Job drawing, mm, ordinate dimensions from the low corner. One solid piece. Give positions to 0.01 mm unless a question says otherwise; leave off trailing zeros. Write each loop counter-clockwise with the first axis right and the second up, starting at its lowest first coordinate (ties: lowest second). Pieces come first, ordered by that corner, then holes. Notation, with made-up numbers: (89.25, 48.25) - (139.25, 48.25) arc R22 cw to (139.25, 71.25) - close; hole circle Ø3 at (15, -37). An arc over 180 degrees is marked (long way). Put each result on its own line as item: value. Start each with the question number.
1. Cut at B-B on z = 65. List the corners of the cut face in (x, y), and give its area (3 significant figures).
2. Drop a flat-ended pin along its axis: pin 1 (4 mm diameter, centred on y = 3.5, z = 53.5, fed in from +X). Give the stop position or say it passes through.
3. Wall check: line 1 (Y direction, x = 0.4, z = 57); line 2 (Z direction, x = 0.35, y = 5.25). Give the ranges that are in metal, low to high.
4. Cut at A-A on x = 0.3. List the corners of the cut face in (y, z), and give its area (3 significant figures).
5. Cut at C-C on y = 6.25. List the corners of the cut face in (x, z), and give its area (3 significant figures).
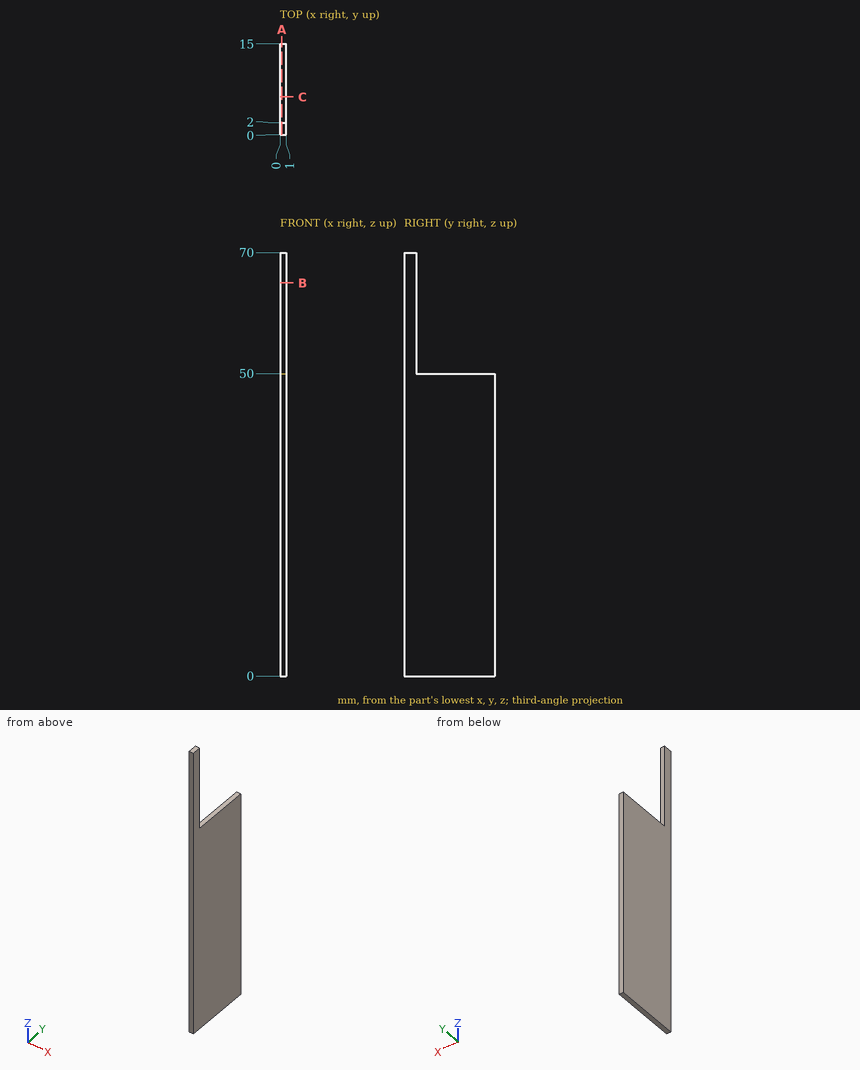
Report:
1. outline: (0, 0) - (1, 0) - (1, 2) - (0, 2) - close
1. area: 2.00 mm²
2. pin 1: stops at x = 1
3. line 1: y = 0 to 2
3. line 2: z = 0 to 50
4. outline: (0, 0) - (15, 0) - (15, 50) - (2, 50) - (2, 70) - (0, 70) - close
4. area: 790 mm²
5. outline: (0, 0) - (1, 0) - (1, 50) - (0, 50) - close
5. area: 50.0 mm²
